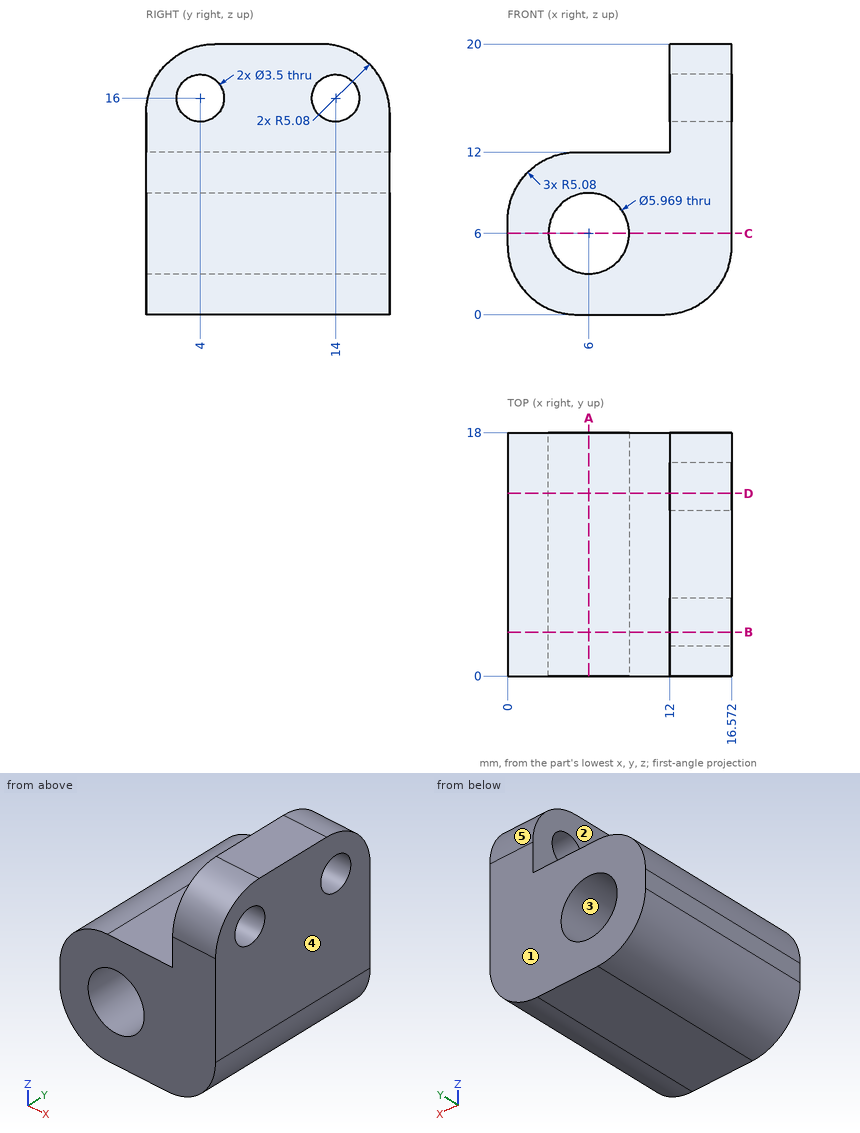
Study the drawing (mm; zero at the part's minimum x, y, z) and answer. A direction names the side the tool comes from. Give positions to 0.01 mm unless a question says otherwise; leave off trailing zeros. Loops run counter-clockwise (first coordinate to the right, second up) from the corner with the lowest first, then second, coordinate; pieces in that order, holes last. Notation, with made-up numbers: (9.5, 79.5) -> (37.5, 79.5) arc R33 ccw to (37.5, 118.5) -> close; hole circle Ø7 at (-11.5, 14). An arc over 180 degrees is marked (long way). Use a Markdown table: item, result. Add a question column.
1) Each of these flat-tipped pins is pushed along its axis until it touches: P1, Ø2, axis at y = 4, z = 16, coming from the -X side; P2, Ø1.5, axis at y = 15.5, z = 15.5, coming from the -X side; P3, Ø1.5, axis at y = 4, z = 10, coming from the -X side; P4, Ø9, axis at y = 7.5, z = 16, coming from the -X side. Where does it stop, or does it pass through?
2) For a pull along Z with two mould halves and no side action, classify the marked faces 3, 4 and 5 as +Z half, -Z half, draft (parallel to the pull), parting line (faces both ways), or undercut.
3) The part is cut by section C-C, the plane z = 6. Determine the outline of the cut face in (x, y), plus the area to 3 significant figures.
4) The part is cut by section A-A, the plane x = 6. Determine the outline of the cut face in (y, z).
5) The part is cut by section B-B, the plane y = 3.25. Determine the outline of the cut face in (x, z).
6) The part is cut by section D-D, the plane y = 13.5. Determine the outline of the cut face in (x, z), plus the area to 3 significant figures.
7) Consider line 1 along X through (y, z) = (12.25, 14); line 2 along X through (y, z) = (14.75, 4.5); line 3 along Z through (x, y) = (15.25, 14). Determine where each line is inside the solid, lowest interval first.
8) Which of the six approach directions +Z, -Z, +X, -X, +Y, -Y give full straight-line access (tool end or side, diameter ignored) to the marked faces 1 and 2?
Reported:
| question | item | result |
|---|---|---|
| 1 | P1 | passes through |
| 1 | P2 | stops at x = 12 |
| 1 | P3 | stops at x = 0.57 |
| 1 | P4 | stops at x = 2.88 |
| 2 | face 3 | undercut |
| 2 | face 4 | draft |
| 2 | face 5 | +Z half |
| 3 | outline | (0, 0) -> (3.02, 0) -> (3.02, 18) -> (0, 18) -> close; (8.98, 0) -> (16.57, 0) -> (16.57, 18) -> (8.98, 18) -> close |
| 3 | area | 191 mm^2 |
| 4 | outline | (0, 0) -> (18, 0) -> (18, 3.02) -> (0, 3.02) -> close; (0, 8.98) -> (18, 8.98) -> (18, 12) -> (0, 12) -> close |
| 5 | outline | (0, 5.08) arc R5.08 ccw to (5.08, 0) -> (11.49, 0) arc R5.08 ccw to (16.57, 5.08) -> (16.57, 14.42) -> (12, 14.42) -> (12, 12) -> (5.08, 12) arc R5.08 ccw to (0, 6.92) -> close; (12, 17.58) -> (16.57, 17.58) -> (16.57, 19.66) -> (12, 19.66) -> close; hole circle Ø5.97 at (6, 6) |
| 6 | outline | (0, 5.08) arc R5.08 ccw to (5.08, 0) -> (11.49, 0) arc R5.08 ccw to (16.57, 5.08) -> (16.57, 14.32) -> (12, 14.32) -> (12, 12) -> (5.08, 12) arc R5.08 ccw to (0, 6.92) -> close; (12, 17.68) -> (16.57, 17.68) -> (16.57, 19.97) -> (12, 19.97) -> close; hole circle Ø5.97 at (6, 6) |
| 6 | area | 175 mm^2 |
| 7 | line 1 | x = 12 to 16.57 |
| 7 | line 2 | x = 0.03 to 3.42, 8.58 to 16.54 |
| 7 | line 3 | z = 1.66 to 14.25, 17.75 to 19.88 |
| 8 | face 1 | +Z, -Z, +X, -X, +Y |
| 8 | face 2 | +Z, -X, +Y, -Y |
